Geometry check sheet. Reference: the model listing, model coordinates, mm. A direction names the side the tool comes from. Round coordinates to 2 decimals unless told otherwise and drop trailing zeros. Loops run counter-clockwise (first coordinate to the right, second up) from the corner with the lowest first, then second, coordinate; pieces in that order, holes last. Notation, with made-up numbers: (2, 82.25) - (30, 82.25) arc R25 cw to (30, 105.25) - close; hole circle Ø9 at (11.5, 74). An arc over 180 degrees is marked (long way). Write item = value, one per line.
```python
from build123d import *

# Parameters (mm, degrees)
EXTRUDE_2_DEPTH                 = 7.5
EXTRUDE_2_DEPTH_BACK            = 7.5
SKETCH_3_W                      = 3
SKETCH_3_H                      = 3
EXTRUDE_3_DEPTH                 = 1
EXTRUDE_4_DEPTH                 = 2
EXTRUDE_4_DEPTH_BACK            = 2
CUT_EXTRUDE_1_REACH             = 10.143
CUT_EXTRUDE_1_DIRECTION_2_REACH = 10.143
FILLET_1_R                      = 0.1


with BuildPart() as part:
    # Sketch 2 → Extrude 2 (new, two sides: drawn at the far end of the back side and taken through both)
    with BuildSketch(Plane.XY.offset(-EXTRUDE_2_DEPTH_BACK)):
        with BuildLine():
            Line((-1.95, -2.5), (-1, -2.5))
            ThreePointArc((-1, -2.5), (-0.861429892, -1.992123498), (-0.484122918, -1.625))
            ThreePointArc((-0.484122918, -1.625), (0, -1), (0.484122918, -1.625))
            ThreePointArc((0.484122918, -1.625), (0.861429892, -1.992123498), (1, -2.5))
            Line((1, -2.5), (1.95, -2.5))
            Line((1.95, -2.5), (1.95, -1.555590279))
            ThreePointArc((1.95, -1.555590279), (1.780042303, -1.088161527), (1.5, -0.677124344))
            Line((1.5, -0.677124344), (1.5, 0))
            Line((1.5, 0), (-1.5, 0))
            Line((-1.5, 0), (-1.5, -0.677124344))
            ThreePointArc((-1.5, -0.677124344), (-1.780042303, -1.088161527), (-1.95, -1.555590279))
            Line((-1.95, -1.555590279), (-1.95, -2.5))
        make_face()
    extrude(amount=EXTRUDE_2_DEPTH + EXTRUDE_2_DEPTH_BACK)

    # Sketch 3 → Extrude 3 (add)
    with BuildSketch(Plane(origin=(0, 0, 0), x_dir=(-1, 0, 0), z_dir=(0, 1, 0))):
        Rectangle(SKETCH_3_W, SKETCH_3_H)
    extrude(amount=EXTRUDE_3_DEPTH)

    # Sketch 4 → Extrude 4 (add, two sides: drawn at the far end of the back side and taken through both)
    with BuildSketch(Plane.XY.offset(-EXTRUDE_4_DEPTH_BACK)):
        with BuildLine():
            Line((-1.95, 2.5), (1.95, 2.5))
            Line((1.95, 2.5), (1.95, 1.555590279))
            ThreePointArc((1.95, 1.555590279), (1.780042303, 1.088161527), (1.5, 0.677124344))
            Line((1.5, 0.677124344), (-1.5, 0.677124344))
            ThreePointArc((-1.5, 0.677124344), (-1.780042303, 1.088161527), (-1.95, 1.555590279))
            Line((-1.95, 1.555590279), (-1.95, 2.5))
        make_face()
    extrude(amount=EXTRUDE_4_DEPTH + EXTRUDE_4_DEPTH_BACK)

    # Sketch 5 → Cut-Extrude 1 (cut, up to next)
    with BuildSketch(Plane(origin=(0, 0, 0), x_dir=(0, 0, -1), z_dir=(1, 0, 0)), mode=Mode.PRIVATE) as cut_extrude_1_sk1:
        with BuildLine():
            Line((1.95, 2.5), (2, 2.5))
            Line((2, 2.5), (2, 0.677124344))
            Line((2, 0.677124344), (1.5, 0.677124344))
            ThreePointArc((1.5, 0.677124344), (1.780042303, 1.088161527), (1.95, 1.555590279))
            Line((1.95, 1.555590279), (1.95, 2.5))
        make_face()
    cut_extrude_1_tool1 = extrude(cut_extrude_1_sk1.sketch, amount=-CUT_EXTRUDE_1_REACH, mode=Mode.PRIVATE) & part.part
    # Sketch 5 → Cut-Extrude 1 (cut, up to next)
    with BuildSketch(Plane(origin=(0, 0, 0), x_dir=(0, 0, -1), z_dir=(1, 0, 0)), mode=Mode.PRIVATE) as cut_extrude_1_sk2:
        with BuildLine():
            Line((-1.95, 2.5), (-1.95, 1.555590279))
            ThreePointArc((-1.95, 1.555590279), (-1.780042303, 1.088161527), (-1.5, 0.677124344))
            Line((-1.5, 0.677124344), (-2, 0.677124344))
            Line((-2, 0.677124344), (-2, 2.5))
            Line((-2, 2.5), (-1.95, 2.5))
        make_face()
    cut_extrude_1_tool2 = extrude(cut_extrude_1_sk2.sketch, amount=-CUT_EXTRUDE_1_REACH, mode=Mode.PRIVATE) & part.part
    add(cut_extrude_1_tool1.solids().sort_by_distance((0, 1.175075, -1.873038))[0], mode=Mode.SUBTRACT)
    add(cut_extrude_1_tool2.solids().sort_by_distance((0, 1.175075, 1.873038))[0], mode=Mode.SUBTRACT)

    # Sketch 5 → Cut-Extrude 1 direction 2 (cut, up to next)
    with BuildSketch(Plane(origin=(0, 0, 0), x_dir=(0, 0, -1), z_dir=(1, 0, 0)), mode=Mode.PRIVATE) as cut_extrude_1_direction_2_sk1:
        with BuildLine():
            Line((1.95, 2.5), (2, 2.5))
            Line((2, 2.5), (2, 0.677124344))
            Line((2, 0.677124344), (1.5, 0.677124344))
            ThreePointArc((1.5, 0.677124344), (1.780042303, 1.088161527), (1.95, 1.555590279))
            Line((1.95, 1.555590279), (1.95, 2.5))
        make_face()
    cut_extrude_1_direction_2_tool1 = extrude(cut_extrude_1_direction_2_sk1.sketch, amount=CUT_EXTRUDE_1_DIRECTION_2_REACH, mode=Mode.PRIVATE) & part.part
    # Sketch 5 → Cut-Extrude 1 direction 2 (cut, up to next)
    with BuildSketch(Plane(origin=(0, 0, 0), x_dir=(0, 0, -1), z_dir=(1, 0, 0)), mode=Mode.PRIVATE) as cut_extrude_1_direction_2_sk2:
        with BuildLine():
            Line((-1.95, 2.5), (-1.95, 1.555590279))
            ThreePointArc((-1.95, 1.555590279), (-1.780042303, 1.088161527), (-1.5, 0.677124344))
            Line((-1.5, 0.677124344), (-2, 0.677124344))
            Line((-2, 0.677124344), (-2, 2.5))
            Line((-2, 2.5), (-1.95, 2.5))
        make_face()
    cut_extrude_1_direction_2_tool2 = extrude(cut_extrude_1_direction_2_sk2.sketch, amount=CUT_EXTRUDE_1_DIRECTION_2_REACH, mode=Mode.PRIVATE) & part.part
    add(cut_extrude_1_direction_2_tool1.solids().sort_by_distance((0, 1.175075, -1.873038))[0], mode=Mode.SUBTRACT)
    add(cut_extrude_1_direction_2_tool2.solids().sort_by_distance((0, 1.175075, 1.873038))[0], mode=Mode.SUBTRACT)

    # Fillet 1
    fillet_1_edges = [part.edges().sort_by_distance(p)[0] for p in [
        (0, 2.5, 1.95),
        (1.95, -2.5, 0),
        (-1.95, -2.5, 0),
        (1.95, 2.5, 0),
        (-1.95, 2.5, 0),
        (0, 2.5, -1.95),
    ]]
    fillet(fillet_1_edges, radius=FILLET_1_R)


solid = part.part
```
(1) Section check A-A (z = 0). Enter the section's corners in (x, y) (3 decimals), then the cut area to 3 significant figures.
Answers follow:
outline = (-1.95, -2.4) arc R0.1 ccw to (-1.85, -2.5) - (-1, -2.5) arc R1 cw to (-0.484, -1.625) arc R0.5 cw (long way) to (0.484, -1.625) arc R1 cw to (1, -2.5) - (1.85, -2.5) arc R0.1 ccw to (1.95, -2.4) - (1.95, -1.556) arc R2 ccw to (1.5, -0.677) - (1.5, 0.677) arc R2 ccw to (1.95, 1.556) - (1.95, 2.4) arc R0.1 ccw to (1.85, 2.5) - (-1.85, 2.5) arc R0.1 ccw to (-1.95, 2.4) - (-1.95, 1.556) arc R2 ccw to (-1.5, 0.677) - (-1.5, -0.677) arc R2 ccw to (-1.95, -1.556) - close
area = 15.6 mm²
(2) Section check B-B (x = -1.25). Enter the section's corners in (y, z).
Answers follow:
outline = (-2.5, -7.5) - (0, -7.5) - (0, -1.5) - (0.68, -1.5) arc R2 ccw to (1.56, -1.95) - (2.4, -1.95) arc R0.1 ccw to (2.5, -1.85) - (2.5, 1.85) arc R0.1 ccw to (2.4, 1.95) - (1.56, 1.95) arc R2 ccw to (0.68, 1.5) - (0, 1.5) - (0, 7.5) - (-2.5, 7.5) - close
(3) Scan lines: L1, parallel to Z at x = 0.45, y = 1.7; L2, parallel to Y at x = -1.35, z = 3.5; L3, parallel to X at y = -1.5, z = -0.25. Record each from-to range of solid material in increasing order. Write a range as [from, to].
Answers follow:
L1 = [-1.95, 1.95]
L2 = [-2.5, 0]
L3 = [-1.94, -0.5], [0.5, 1.94]
(4) Set-up check for faces 1 (the flat face through (1.5, 0, 0)), 2 (the flat face through (-1.5, 0, 0)), 3 (the cylindrical face through (-0.865, -1.999, -0.105)), 4 (the flat face through (0, 2, 1.95)), 5 (the flat face through (1.95, -2, 0)): record each of +Z, -Z, +X, -X, +Y, -Y from which the full face is reachable in a straight line by a thin tool's end or side.
Answers follow:
face_1 = +Z, -Z, +X
face_2 = +Z, -Z, -X
face_3 = +Z, -Z, -Y
face_4 = +Z, +X, -X, +Y
face_5 = +Z, -Z, +X, +Y, -Y
(5) Gauge pin test, flat ends, axial feed: pin 1 (0.9 mm diameter, centred on x = 0.5, y = 2, fed in from +Z); pin 2 (2 mm diameter, centred on y = 0, z = -1.5, fed in from +X); pin 3 (1.1 mm diameter, centred on y = 0, z = -2.5, fed in from +X). Record the tip position at first contact, or that the pin passes through.
Answers follow:
pin_1 = 1.95
pin_2 = 1.73
pin_3 = 1.5
(6) Section check D-D (y = 1.85). Enter the section's corners in (x, z).
Answers follow:
outline = (-1.95, -1.95) - (1.95, -1.95) - (1.95, 1.95) - (-1.95, 1.95) - close
(7) Section check C-C (y = -1.85). Enter the section's corners in (x, z), then the cut area to 3 significant figures.
Answers follow:
outline = (-1.95, -7.5) - (-0.76, -7.5) - (-0.76, 7.5) - (-1.95, 7.5) - close; (0.76, -7.5) - (1.95, -7.5) - (1.95, 7.5) - (0.76, 7.5) - close
area = 35.7 mm²
